Build history of the part. All positions in model axes, mm. Round coordinates to 2 decimals unless told otherwise and drop trailing zeros. Write each loop counter-clockwise with the first axis right and the second up, starting at its lowest first coordinate (ties: lowest second). Pieces come first, ordered by that corner, then holes. Notation, with made-up numbers: (31, 87) - (64, 87) arc R21 ccw to (64, 122) - close; hole circle Ø4 at (-18.75, 13.5). An arc over 180 degrees is marked (long way). Write each question's results on one line, items separated by ' | '.
Autodesk Inventor part; units mm, degrees
ref_plane "YZ Plane" through (0, 0, 0) normal (1, 0, 0) x (0, 1, 0)
ref_plane "XZ Plane" through (0, 0, 0) normal (0, 1, 0) x (-1, 0, 0)
ref_plane "XY Plane" through (0, 0, 0) normal (0, 0, 1) x (1, 0, 0)
sketch "Sketch1" plane through (0, 0, 0) normal (0, 1, 0) x (-1, 0, 0)
  line L0 (-988.9153, -1793.2204) -> (194.3412, -1476.1678)
  line L1 (189.3384, -1438.1678) -> (5.0028, -38)
  line L2 (-998.7504, -1756.5152) -> (-1225.2435, -36.1295)
  line L3 (-961.7285, -1746.5952) -> (152.3165, -1448.0878)
  line L4 (152.3165, -1448.0878) -> (-33.3251, -38)
  line L5 (-33.3251, -38) -> (-1186.6693, -38)
  line L6 (-961.7285, -1746.5952) -> (-1186.6693, -38)
  line L7 (-998.7504, -1756.5152) -> (-988.9153, -1793.2204)
  line L8 (-1225.2435, -36.1295) -> (-1225.2435, 0)
  line L9 (189.3384, -1438.1678) -> (199.1735, -1474.873)
  line L10 (194.3412, -1476.1678) -> (199.1735, -1474.873)
  line L11 (5.0028, -38) -> (5.0028, 0)
  line L12 (5.0028, 0) -> (-1225.2435, 0)
  dimension "d7" = 38
  dimension "d8" = 38
extrude "Extrusion1" add sketch "Sketch1" along normal blind 114
sketch "Sketch2" plane through (0, 114, 0) normal (0, 1, 0) x (1, 0, 0)
  line L0 (33.3251, 38) -> (-152.3165, 1448.0878)
  line L1 (-189.3384, 1438.1678) -> (-5.0028, 38)
  line L2 (-5.0028, 38) -> (-5.0028, 0)
  line L3 (998.7504, 1756.5152) -> (988.9153, 1793.2204)
  line L4 (-152.3165, 1448.0878) -> (-189.3384, 1438.1678)
  line L5 (33.3251, 38) -> (-5.0028, 38)
  point P0 (0, 0)
extrude "Extrusion2" cut sketch "Sketch2" against normal blind 1
sketch "Sketch4" plane through (0, 114, 0) normal (0, 1, 0) x (1, 0, 0)
  line L0 (961.7285, 1746.5952) -> (1186.6693, 38)
  line L1 (1225.2435, 0) -> (1225.2435, 36.1295)
  line L2 (1225.2435, 36.1295) -> (998.7504, 1756.5152)
  line L3 (-199.1735, 1474.873) -> (-189.3384, 1438.1678)
  line L4 (961.7285, 1746.5952) -> (998.7504, 1756.5152)
  line L5 (1186.6693, 38) -> (1224.9972, 38)
  point P0 (0, 0)
extrude "Extrusion4" cut sketch "Sketch4" against normal blind 1
properties part number "panelDframe" material "Wood (Cherry)"
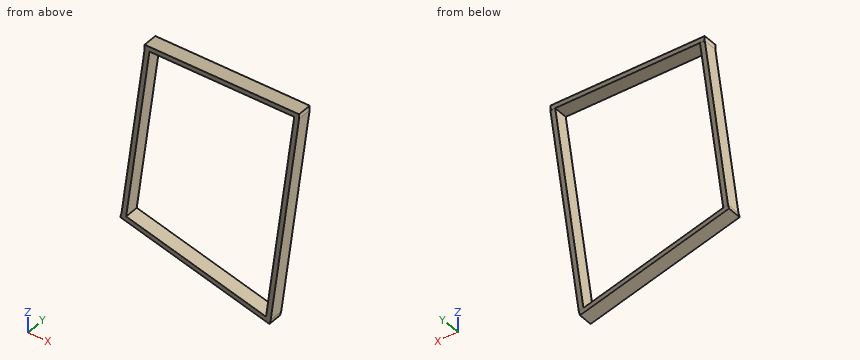
(1) Slice it at A-A, the plane y = 25.5. Write the cut outline in (x, z), and give its area (3 significant figures).
Worked answers:
outline: (-199.17, -1474.87) - (-194.34, -1476.17) - (988.92, -1793.22) - (998.75, -1756.52) - (1225.24, -36.13) - (1225.24, 0) - (-5, 0) - (-5, -38) - (-189.34, -1438.17) - close; hole (-152.32, -1448.09) - (961.73, -1746.6) - (1186.67, -38) - (33.33, -38) - close | area: 213,000 mm2
(2) Slice it at B-B, the plane z = -1003.5. Write the cut outline in (x, y).
Worked answers:
outline: (-132.11, 0) - (-93.79, 0) - (-93.79, 113) - (-132.11, 113) - close; (1059.56, 0) - (1097.89, 0) - (1097.89, 113) - (1059.56, 113) - close
(3) Drill centre lines: probe 1 along X at (y, z) = (27.5, -293.5); probe 2 along Z at (x, y) = (914, 57); probe 3 along X at (y, z) = (96, -1330). Where is each one in solid material? Low to high. Write a range as [from, to].
Worked answers:
probe 1: x = [-38.64, -0.31], [1153.03, 1191.36] | probe 2: z = [-1773.15, -1733.81], [-38, 0] | probe 3: x = [-175.1, -136.77], [1016.57, 1054.9]
(4) Flat gauge pins, fed straight in: pin 1 Ø5 at (y, z) = (25.5, -980) entering from -X; pin 2 Ø3 at (x, z) = (-1, -225) entering from +Y; pin 3 Ø5 at (y, z) = (29.5, -1031) entering from -X. Where does each tip first touch, or does it go through?
Worked answers:
pin 1: stops at x = -129.35 | pin 2: stops at y = 113 | pin 3: stops at x = -136.06
(5) Slice it at C-C, the plane x = 686. Write the cut outline in (y, z).
Worked answers:
outline: (0, -1712.05) - (114, -1712.05) - (114, -1672.71) - (0, -1672.71) - close; (0, -38) - (114, -38) - (114, 0) - (0, 0) - close
